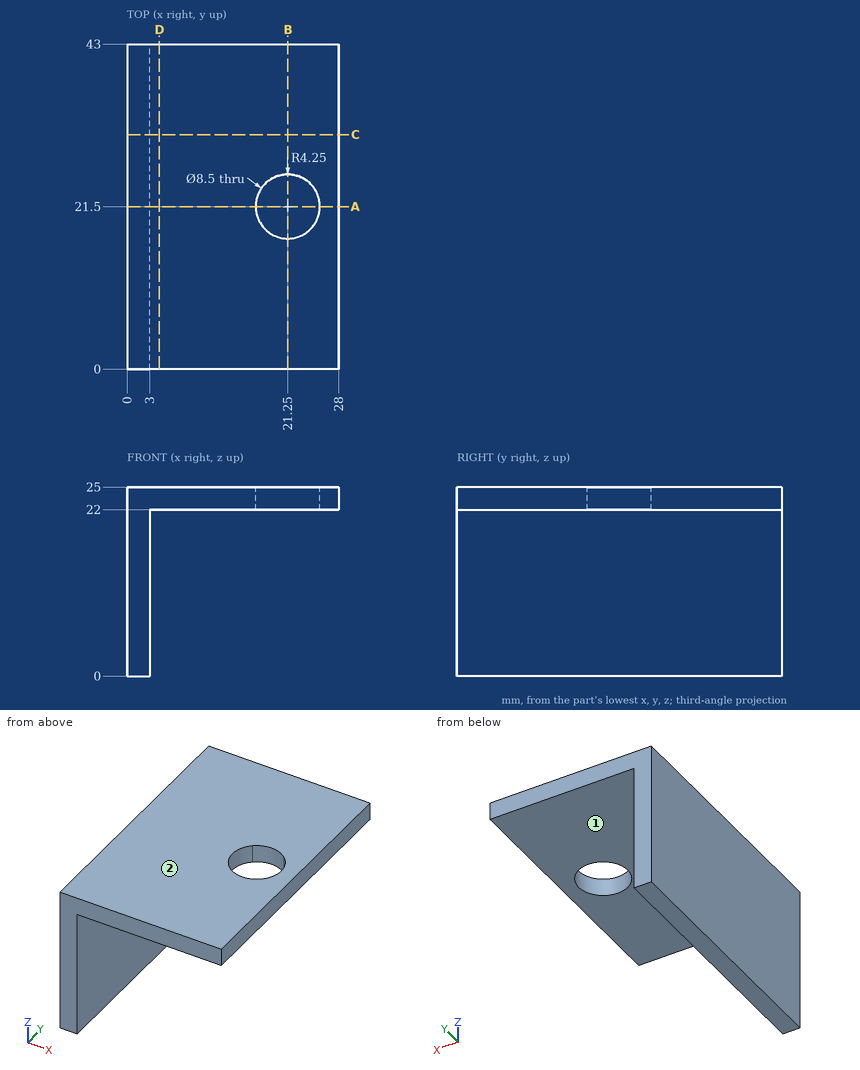
For this review, use the dimensioned drawing (mm, ordinates from the lowest corner) and the shaded views. A direction names the side the tool comes from. Give positions to 0.01 mm unless a question says otherwise; leave off trailing zeros. Order: outer loops, then holes, each group sorted by start corner. A loop starts at its lowest first (then second) coordinate and runs counter-clockwise, first axis right, second up. Notation, with made-up numbers: (56.25, 29) - (95.25, 29) arc R24 ccw to (95.25, 51) - close; hole circle Ø4 at (-33.75, 84). An arc over 180 degrees is marked (long way). Use CSV: the item, a comma, the result in double quotes. Start each with the question number.
Q1. To check wall thickness, follow line 1 along X through (y, z) = (21.5, 23.05); line 2 along Y through (x, z) = (21.25, 22.9); line 3 along Z through (x, y) = (5, 37.5). State the ranges of each line that lie inside material, in increasing order. Write a range as [from, to].
Q2. We need section A-A, the plane y = 21.5. Write out the cut boundary in (x, z), and give its area (4 significant figures).
Q3. Clearance check with flat-ended pins moving along their axes: pin 1 Ø6.5 at (y, z) = (17, 13.5) entering from +X; pin 2 Ø2 at (x, y) = (6.5, 15.5) entering from -Z. State where each tip first meets the part, or that it passes through.
Q4. We need section D-D, the plane x = 4.25. Write out the cut boundary in (y, z).
Q5. We need section B-B, the plane x = 21.25. Write out the cut boundary in (y, z).
Q6. We need section C-C, the plane y = 31. Write out the cut boundary in (x, z), and give its area (3 significant figures).
Q7. Tool access review of the marked faces 1 and 2: name each direction out of +Z, -Z, +X, -X, +Y, -Y from which nothing blocks a thin tool from reaching the whole face with its end or side.
Outcome:
1,line 1,"x = [0, 17], [25.5, 28]"
1,line 2,"y = [0, 17.25], [25.75, 43]"
1,line 3,"z = [22, 25]"
2,outline,"(0, 0) - (3, 0) - (3, 22) - (17, 22) - (17, 25) - (0, 25) - close; (25.5, 22) - (28, 22) - (28, 25) - (25.5, 25) - close"
2,area,"124.5 mm^2"
3,pin 1,"stops at x = 3"
3,pin 2,"stops at z = 22"
4,outline,"(0, 22) - (43, 22) - (43, 25) - (0, 25) - close"
5,outline,"(0, 22) - (17.25, 22) - (17.25, 25) - (0, 25) - close; (25.75, 22) - (43, 22) - (43, 25) - (25.75, 25) - close"
6,outline,"(0, 0) - (3, 0) - (3, 22) - (28, 22) - (28, 25) - (0, 25) - close"
6,area,"150 mm^2"
7,face 1,"-Z, +X, +Y, -Y"
7,face 2,"+Z, +X, -X, +Y, -Y"
